Here's the drawing with two shaded views (mm, measured from the low corner). I have some questions. Give positions to 0.01 mm unless a question says otherwise; leave off trailing zeros. Order: outer loops, then holes, each group sorted by start corner. A loop starts at its lowest first (then second) coordinate and runs counter-clockwise, first axis right, second up. Notation, with made-up numbers: M 76.25,-11 L 109.25,-11 A18 cw 109.25,23 Z; hole C 67.25,-20 d7. An arc over 180 degrees is marked long. Write each question's results on one line, items separated by ' | '.
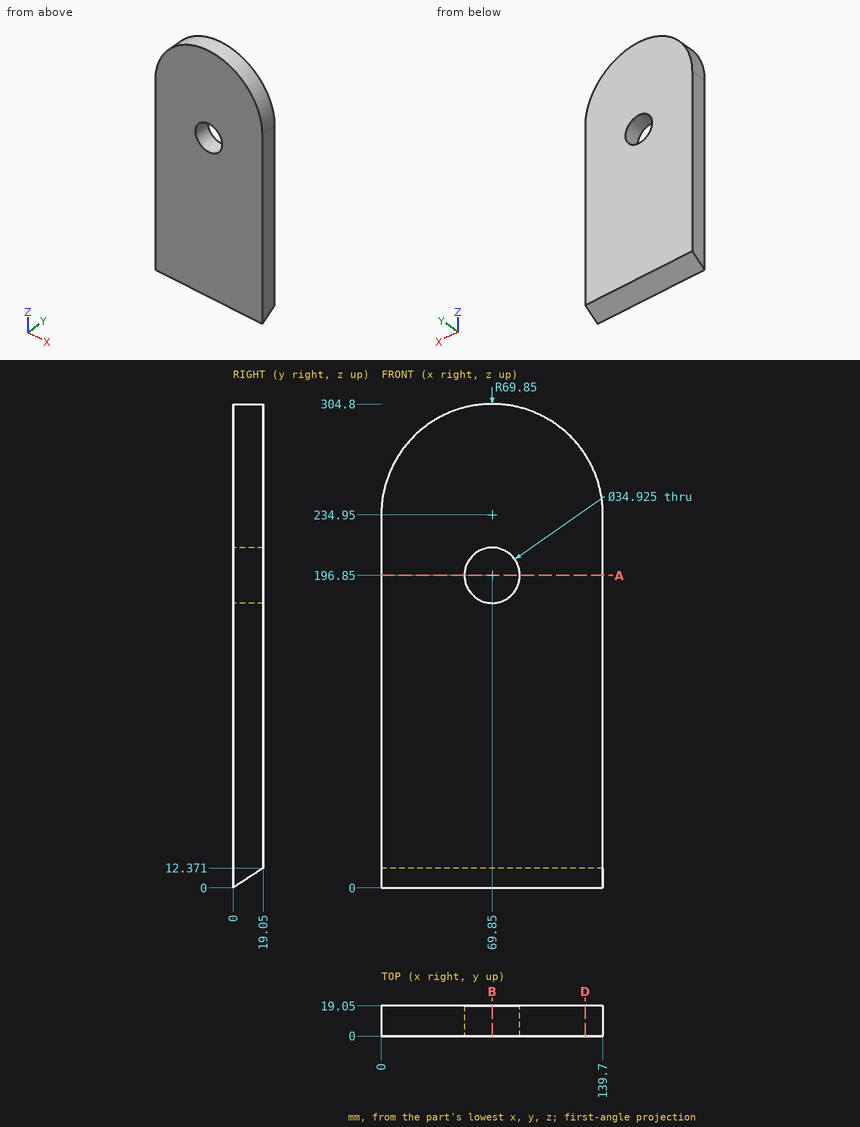
(1) Imagine slicing it at A-A, the plane z = 196.85. Write out the boundary of the cut face in (x, y).
Data:
outline: M 0,0 L 52.39,0 L 52.39,19.05 L 0,19.05 Z; M 87.31,0 L 139.7,0 L 139.7,19.05 L 87.31,19.05 Z
(2) Imagine slicing it at D-D, the plane x = 128.5. Write out the boundary of the cut face in (y, z).
Data:
outline: M 0,0 L 19.05,12.37 L 19.05,272.89 L 0,272.89 Z
(3) I need wall thicknesses on L1, parallel to Z at x = 66.5, y = 14; L2, parallel to Z at x = 69.85, y = 11; L3, parallel to Z at x = 12, y = 7.25 (1 decimal). Which ranges of each line are inside material? Lowest first, please. Write a range as from..to.
Data:
L1: z = 9.09..179.71, 213.99..304.72 | L2: z = 7.14..179.39, 214.31..304.8 | L3: z = 4.7..274.1
(4) Will these pins go through, and if not, where does the flat tip stop? P1, Ø2, axis at x = 96.5, z = 137, coming from the -Y side; P2, Ø1, axis at x = 109.5, y = 14.5, coming from the +Z side; P3, Ø8, axis at y = 5.5, z = 266.5, coming from the -X side.
Data:
P1: stops at y = 0 | P2: stops at z = 292.8 | P3: stops at x = 5.66
(5) Imagine slicing it at B-B, the plane x = 69.85. Write out the boundary of the cut face in (y, z), plus the area to 3 significant figures.
Data:
outline: M 0,0 L 19.05,12.37 L 19.05,179.39 L 0,179.39 Z; M 0,214.31 L 19.05,214.31 L 19.05,304.8 L 0,304.8 Z | area: 5,020 mm2
